Part model, mm, in its own coordinate system. A direction names the side the tool comes from. Round coordinates to 2 decimals unless told otherwise and drop trailing zeros. Order: outer loops, then holes, each group sorted by start corner. A loop starts at its lowest first (then second) coordinate and runs counter-clockwise, first axis right, second up. Notation, with made-up numbers: (52.25, 89) - (76.25, 89) arc R20 ccw to (76.25, 100) - close; hole circle Ø1 at (23, -24.5). An arc over 180 degrees is marked (long way). Answer as a JSON object with one key per item and string values.
```python
from build123d import *

# Parameters (mm, degrees)
SKETCH3_W = 0.254
SKETCH3_H = 0.508


with BuildPart() as part:
    # Sketch1 → Revolve1 (revolve)
    with BuildSketch(Plane.XY):
        Polygon((0, 0), (0, 3.175), (294.4876, 3.175), (294.4876, 9.62025), (315.9252, 9.62025), (315.9252, 0), align=None)
    revolve(axis=Axis((315.9252, 0, 0), (-1, 0, 0)))

    # Sketch2 → Revolve2 (revolve)
    with BuildSketch(Plane.XY):
        Polygon((-12.7, 0), (-12.7, 2.63398), (-12.15898, 3.175), (0, 3.175), (0, 0), align=None)
    revolve(axis=Axis((0, 0, 0), (-1, 0, 0)))

    # Sketch3 → Cut-Revolve1 (revolve, cut)
    with BuildSketch(Plane.XY):
        with Locations((-0.127, 3.175)):
            Rectangle(SKETCH3_W, SKETCH3_H)
    revolve(axis=Axis((0, 0, 0), (-1, 0, 0)), mode=Mode.SUBTRACT)


solid = part.part
```
Item 1: Tool access for faces 1 (the cylindrical face through (-6.12, -0.69, 3.1)), 2 (the cylindrical face through (305.36, -2.09, 9.39)): list every direction of +Z, -Z, +X, -X, +Y, -Y with a clear straight run to the whole face (end or side of a thin tool).
Taken from the geometry:
{"face 1": "-X", "face 2": "+X, -X"}
Item 2: Probe L1, parallel to X at y = -1.5, z = -3.25; L2, parallel to Y at x = 10, z = -1.75; L3, parallel to Z at x = 232.5, y = -1.5. List the from-to ranges inside material, lowest first. Write a range as from..to.
Taken from the geometry:
{"L1": "294.49..315.93", "L2": "-2.65..2.65", "L3": "-2.8..2.8"}
Item 3: Drop flat-ended pins along their axis: P1, Ø10, axis at x = 229, y = 3, coming from the +Z side (3 decimals); P2, Ø1, axis at x = 247.5, z = 1.5, coming from the +Y side; P3, Ø6, axis at y = -4, z = 7.5, coming from the -X side. Give the stop position or say it passes through.
Taken from the geometry:
{"P1": "z = 3.175", "P2": "y = 3.01", "P3": "x = 294.49"}
Item 4: Cut at A-A (x = 25.5). Write the cut outline in (y, z) (3 decimals), plus the area to 3 significant figures.
Taken from the geometry:
{"outline": "circle Ø6.35 at (0, 0)", "area": "31.7 mm2"}
Item 5: Cut at B-B (z = -6). Write the cut outline in (x, y), plus the area to 3 significant figures.
Taken from the geometry:
{"outline": "(294.49, -7.52) - (315.93, -7.52) - (315.93, 7.52) - (294.49, 7.52) - close", "area": "322 mm2"}
